Autodesk Inventor part; units mm, degrees
ref_plane "YZ Plane" through (0, 0, 0) normal (1, 0, 0) x (0, 1, 0)
ref_plane "XZ Plane" through (0, 0, 0) normal (0, 1, 0) x (-1, 0, 0)
ref_plane "XY Plane" through (0, 0, 0) normal (0, 0, 1) x (1, 0, 0)
sketch "Sketch1" plane through (0, 0, 0) normal (0, 1, 0) x (-1, 0, 0)
  line L0 (15.8278, -0.0229) -> (15.8278, 14.2578)
  arc A0 (15.8278, 14.2578) -> (10.4826, 16.0171) centre (10.4826, 7.0171) ccw
  line L1 (10.4826, 16.0171) -> (4.0229, 16.0171)
  arc A1 (0.0229, 18.0171) -> (4.0229, 16.0171) centre (4.0229, 21.0171) ccw
  line L2 (0.0229, 18.0171) -> (15.8278, 18.0171)
  line L3 (15.8278, 18.0171) -> (15.8278, 18.7671)
  line L4 (15.8278, 18.7671) -> (15.6604, 19.2271)
  line L5 (15.6604, 19.2271) -> (14.9004, 19.2271)
  line L6 (14.9004, 19.2271) -> (14.7329, 18.7671)
  line L7 (14.7329, 18.7671) -> (13.7978, 18.7671)
  line L8 (13.7978, 18.7671) -> (13.6304, 19.2271)
  line L9 (13.6304, 19.2271) -> (12.8704, 19.2271)
  line L10 (12.8704, 19.2271) -> (12.7029, 18.7671)
  line L11 (12.7029, 18.7671) -> (11.7678, 18.7671)
  line L12 (11.7678, 18.7671) -> (11.6004, 19.2271)
  line L13 (11.6004, 19.2271) -> (10.8404, 19.2271)
  line L14 (10.8404, 19.2271) -> (10.6729, 18.7671)
  line L15 (10.6729, 18.7671) -> (9.7378, 18.7671)
  line L16 (9.7378, 18.7671) -> (9.5704, 19.2271)
  line L17 (9.5704, 19.2271) -> (8.8104, 19.2271)
  line L18 (8.8104, 19.2271) -> (8.6429, 18.7671)
  line L19 (8.6429, 18.7671) -> (7.7078, 18.7671)
  line L20 (7.7078, 18.7671) -> (7.5404, 19.2271)
  line L21 (7.5404, 19.2271) -> (6.7804, 19.2271)
  line L22 (6.7804, 19.2271) -> (6.6129, 18.7671)
  line L23 (6.6129, 18.7671) -> (5.6778, 18.7671)
  line L24 (5.6778, 18.7671) -> (5.5104, 19.2271)
  line L25 (5.5104, 19.2271) -> (4.7504, 19.2271)
  line L26 (4.7504, 19.2271) -> (4.5829, 18.7671)
  line L27 (4.5829, 18.7671) -> (3.6478, 18.7671)
  line L28 (3.6478, 18.7671) -> (3.4804, 19.2271)
  line L29 (3.4804, 19.2271) -> (2.7204, 19.2271)
  line L30 (2.7204, 19.2271) -> (2.5529, 18.7671)
  line L31 (2.5529, 18.7671) -> (1.6178, 18.7671)
  line L32 (1.6178, 18.7671) -> (1.4504, 19.2271)
  line L33 (1.4504, 19.2271) -> (0.6904, 19.2271)
  line L34 (0.6904, 19.2271) -> (0.5229, 18.7671)
  line L35 (0.5229, 18.7671) -> (0.0229, 18.7671)
  line L36 (0.0229, 18.7671) -> (0.0229, 20.2271)
  arc A2 (5.0229, 25.2271) -> (0.0229, 20.2271) centre (5.0229, 20.2271) ccw
  line L37 (5.0229, 25.2271) -> (14.0269, 25.2271)
  line L38 (14.0269, 25.2271) -> (14.9274, 25.2583)
  line L39 (14.9274, 25.2583) -> (15.8278, 25.4494)
  line L40 (15.8278, 25.4494) -> (15.8278, 63.4771)
  line L41 (15.8278, 63.4771) -> (79.3278, 63.4771)
  line L42 (79.3278, 63.4771) -> (79.3278, 50.4494)
  line L43 (79.3278, 50.4494) -> (80.2012, 50.261)
  line L44 (80.2012, 50.261) -> (81.1287, 50.2271)
  line L45 (81.1287, 50.2271) -> (90.1326, 50.2271)
  arc A3 (95.1326, 45.2271) -> (90.1326, 50.2271) centre (90.1326, 45.2271) ccw
  line L46 (95.1326, 45.2271) -> (95.1326, 43.7671)
  line L47 (95.1326, 43.7671) -> (94.6326, 43.7671)
  line L48 (94.6326, 43.7671) -> (94.4652, 44.2271)
  line L49 (94.4652, 44.2271) -> (93.7052, 44.2271)
  line L50 (93.7052, 44.2271) -> (93.5378, 43.7671)
  line L51 (93.5378, 43.7671) -> (92.6026, 43.7671)
  line L52 (92.6026, 43.7671) -> (92.4352, 44.2271)
  line L53 (92.4352, 44.2271) -> (91.6752, 44.2271)
  line L54 (91.6752, 44.2271) -> (91.5078, 43.7671)
  line L55 (91.5078, 43.7671) -> (90.5726, 43.7671)
  line L56 (90.5726, 43.7671) -> (90.4052, 44.2271)
  line L57 (90.4052, 44.2271) -> (89.6452, 44.2271)
  line L58 (89.6452, 44.2271) -> (89.4778, 43.7671)
  line L59 (89.4778, 43.7671) -> (88.5426, 43.7671)
  line L60 (88.5426, 43.7671) -> (88.3752, 44.2271)
  line L61 (88.3752, 44.2271) -> (87.6152, 44.2271)
  line L62 (87.6152, 44.2271) -> (87.4478, 43.7671)
  line L63 (87.4478, 43.7671) -> (86.5126, 43.7671)
  line L64 (86.5126, 43.7671) -> (86.3452, 44.2271)
  line L65 (86.3452, 44.2271) -> (85.5852, 44.2271)
  line L66 (85.5852, 44.2271) -> (85.4178, 43.7671)
  line L67 (85.4178, 43.7671) -> (84.4826, 43.7671)
  line L68 (84.4826, 43.7671) -> (84.3152, 44.2271)
  line L69 (84.3152, 44.2271) -> (83.5552, 44.2271)
  line L70 (83.5552, 44.2271) -> (83.3878, 43.7671)
  line L71 (83.3878, 43.7671) -> (82.4526, 43.7671)
  line L72 (82.4526, 43.7671) -> (82.2852, 44.2271)
  line L73 (82.2852, 44.2271) -> (81.5252, 44.2271)
  line L74 (81.5252, 44.2271) -> (81.3578, 43.7671)
  line L75 (81.3578, 43.7671) -> (80.4226, 43.7671)
  line L76 (80.4226, 43.7671) -> (80.2552, 44.2271)
  line L77 (80.2552, 44.2271) -> (79.4952, 44.2271)
  line L78 (79.4952, 44.2271) -> (79.3278, 43.7671)
  line L79 (79.3278, 43.7671) -> (79.3278, 43.0171)
  line L80 (79.3278, 43.0171) -> (95.1326, 43.0171)
  arc A4 (91.1326, 41.0171) -> (95.1326, 43.0171) centre (91.1326, 46.0171) ccw
  line L81 (91.1326, 41.0171) -> (84.673, 41.0171)
  arc A5 (84.673, 41.0171) -> (79.3278, 39.2578) centre (84.673, 32.0171) ccw
  line L82 (79.3278, 39.2578) -> (79.3278, -0.0229)
  line L83 (79.3278, -0.0229) -> (66.6278, -0.0229)
  line L84 (66.6278, -0.0229) -> (66.6278, 50.7771)
  line L85 (66.6278, 50.7771) -> (28.5278, 50.7771)
  line L86 (28.5278, 50.7771) -> (28.5278, -0.0229)
  line L87 (28.5278, -0.0229) -> (15.8278, -0.0229)
  circle A6 centre (22.1778, 5.9146) radius 1.75
  circle A7 centre (22.1778, 57.5396) radius 1.75
  circle A8 centre (72.9778, 57.5396) radius 1.75
  circle A9 centre (72.9778, 5.9146) radius 1.75
  point P0 (0, 0)
extrude "Extrusion1" add sketch "Sketch1" along normal blind 4.5
properties part number "x carriage belt tensioner"
For this review, take the finished solid that the model builds, in its own axes (mm). A direction names the side the tool comes from. Give positions to 0.01 mm unless a question says otherwise; leave off trailing zeros. Loops run counter-clockwise (first coordinate to the right, second up) from the corner with the lowest first, then second, coordinate; pieces in that order, holes last. Notation, with made-up numbers: (29, 63) - (76, 63) arc R19 ccw to (76, 83) - close; hole circle Ø10 at (14.5, 15.5). An arc over 180 degrees is marked (long way). Write each question's results on one line, items separated by ' | '.
(1) For line 1 along X through (y, z) = (2.45, 33.5); line 2 along X through (y, z) = (1.2, 57); line 3 along X through (y, z) = (3.45, 20.5), list the stretches that pass through material, from the lowest coordinate up.
Conclusion:
line 1: -79.33 to -66.63, -28.53 to -15.83 | line 2: -79.33 to -74.64, -71.31 to -23.84, -20.51 to -15.83 | line 3: -79.33 to -66.63, -28.53 to -0.03
(2) Draft analysis for pull direction X (two halves, no side actions). For faces 5 (the cylindrical face through (-23.794, 2.218, 6.585)), 6 (the cylindrical face through (-13.258, 2.218, 15.578)), 7 (the flat face through (-86, 2, 50.227)), state which applies: +X half, -X half, draft (parallel to the pull), parting line (faces both ways), or undercut.
Conclusion:
face 5: undercut | face 6: +X half | face 7: draft
(3) For faces 1 (the flat face through (-87, 2, 43.017)), 2 (the flat face through (-15.828, 2, 44)), 3 (the flat face through (-79.328, 2, 57)), 4 (the flat face through (-66.628, 2, 25)), list the 3-axis set-ups (+Z, -Z, +X, -X, +Y, -Y) from which the entire face can be reached by the end or side of a thin tool; tool diameter is ignored.
Conclusion:
face 1: -X, +Y, -Y | face 2: +Z, +X, +Y, -Y | face 3: +Z, -X, +Y, -Y | face 4: -Z, +Y, -Y
(4) Take a section at B-B (y = 2.15). State how many separate pieces and enclosed holes the cut face has, then the cut area to 3 significant figures.
Conclusion:
separate pieces: 1 | enclosed holes: 4 | area: 2,310 mm^2
(5) Take a section at A-A (z = 27.5). Give the boundary of the cut face in (x, y).
Conclusion:
outline: (-79.33, 0) - (-66.63, 0) - (-66.63, 4.5) - (-79.33, 4.5) - close; (-28.53, 0) - (-15.83, 0) - (-15.83, 4.5) - (-28.53, 4.5) - close
(6) Take a section at C-C (x = -42). Give the boundary of the cut face in (y, z).
Conclusion:
outline: (0, 50.78) - (4.5, 50.78) - (4.5, 63.48) - (0, 63.48) - close
(7) For pin 1 Ø2 at (x, y) = (-45, 2) entering from -Z; pin 2 Ø0.8 at (x, y) = (-88, 3) entering from -Z; pin 3 Ø2 at (y, z) = (0.5, 7.5) entering from -X; pin 4 Ø2 at (x, z) = (-22.18, 5.91) entering from -Y, all flat-tipped, find the tip position at first contact; note any pin that passes through.
Conclusion:
pin 1: z = 50.78 | pin 2: z = 41.02 | pin 3: x = -79.33 | pin 4: through
